from build123d import *

# Parameters (mm, degrees)
F2_DEPTH = 4
F3_DEPTH = 25


with BuildPart() as f2:
    # F0 (on Top) → F2 (new body)
    with BuildSketch(Plane.XY):
        with BuildLine():
            Line((40, 8), (0, 8))
            ThreePointArc((0, 8), (-6, 2), (0, -4))
            Line((0, -4), (40, -4))
            ThreePointArc((40, -4), (46, 2), (40, 8))
        make_face()
    extrude(amount=F2_DEPTH)

    # F1 (on Top) → F3 (cut)
    with BuildSketch(Plane.XY):
        with BuildLine():
            ThreePointArc((0, 4), (-2, 2), (0, 0))
            Line((0, 0), (40, 0))
            ThreePointArc((40, 0), (42, 2), (40, 4))
            Line((40, 4), (0, 4))
        make_face()
    extrude(amount=F3_DEPTH, mode=Mode.SUBTRACT)


solid = f2.part
CAD build for the part. Positions are in the model's coordinates, mm. A direction names the side the tool comes from. Round coordinates to 2 decimals unless told otherwise and drop trailing zeros. Order: outer loops, then holes, each group sorted by start corner. A loop starts at its lowest first (then second) coordinate and runs counter-clockwise, first axis right, second up. Notation, with made-up numbers: (76.25, 60.25) - (83.25, 60.25) arc R21 cw to (83.25, 82.25) - close; hole circle Ø9 at (1.5, 1). An arc over 180 degrees is marked (long way). Return JSON: item names as keys, results as strings.
(1) Cut at A-A (y = 2). Give the cut face in (x, z), then the cut area to 3 significant figures.
Answer key:
{"outline": "(-6, 0) - (-2, 0) - (-2, 4) - (-6, 4) - close; (42, 0) - (46, 0) - (46, 4) - (42, 4) - close", "area": "32.0 mm^2"}
(2) Cut at C-C (z = 2.7). Give the cut face in (x, y), then the cut area to 3 significant figures.
Answer key:
{"outline": "(0, -4) - (40, -4) arc R6 ccw to (40, 8) - (0, 8) arc R6 ccw to start; hole (0, 0) - (40, 0) arc R2 ccw to (40, 4) - (0, 4) arc R2 ccw to start", "area": "421 mm^2"}
(3) Cut at B-B (x = 9). Give the cut face in (y, z).
Answer key:
{"outline": "(-4, 0) - (0, 0) - (0, 4) - (-4, 4) - close; (4, 0) - (8, 0) - (8, 4) - (4, 4) - close"}
(4) Pin check, flat tips, straight feed: pin 1 Ø1.5 at (x, y) = (12.5, 2) entering from -Z; pin 2 Ø1.5 at (y, z) = (-2.5, 3) entering from +X. Stop position of each tip, or through.
Answer key:
{"pin 1": "passes through", "pin 2": "stops at x = 44.68"}
(5) Cut at D-D (y = 6.75). Give the cut face in (x, z).
Answer key:
{"outline": "(-3.67, 0) - (43.67, 0) - (43.67, 4) - (-3.67, 4) - close"}
(6) Wall check: probe 1 along Y at (x, z) = (20, 3.05); probe 2 along X at (y, z) = (2.5, 2.2); probe 3 along X at (y, z) = (3.25, 3.65). Give the ranges that are in metal, low to high. Write a range as from..to.
Answer key:
{"probe 1": "y = -4..0, 4..8", "probe 2": "x = -5.98..-1.94, 41.94..45.98", "probe 3": "x = -5.87..-1.56, 41.56..45.87"}
(7) Tool access for faces 1 (the face through (20, 4, 2)), 2 (the face through (20, 8, 2)): list every direction of +Z, -Z, +X, -X, +Y, -Y with a clear straight run to the whole face (end or side of a thin tool).
Answer key:
{"face 1": "+Z, -Z", "face 2": "+Z, -Z, +X, -X, +Y"}
(8) Pull direction Y, two halves, no side cores. Call faces 3 (the face through (20, 0, 2)), 4 (the face through (20, -1, 0)), 5 (the face through (-2, 2, 2)), 6 (the face through (46, 2, 2)): +Y half, -Y half, draft (parallel to the pull), parting line (faces both ways), or undercut.
Answer key:
{"face 3": "undercut", "face 4": "draft", "face 5": "undercut", "face 6": "parting line"}
